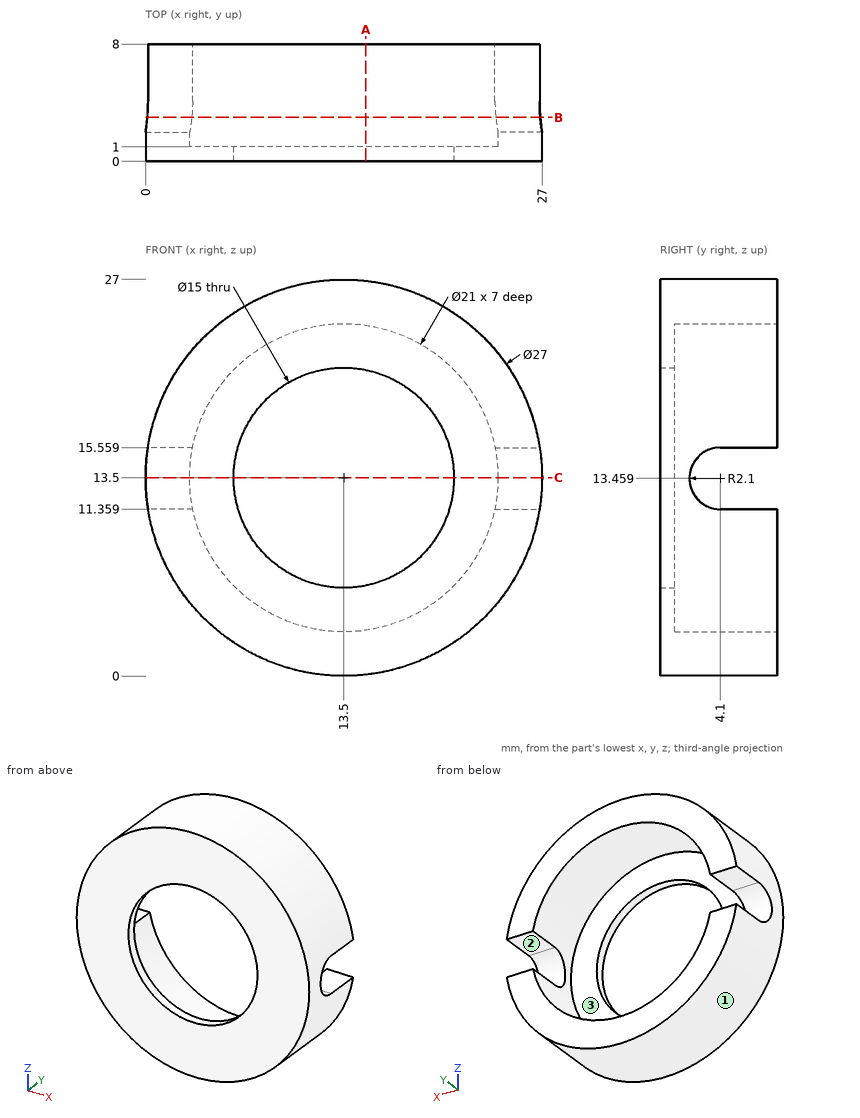
Input: dimensioned drawing with shaded views. Units: mm. Origin: part minimum x, y, z. A direction names the side the tool comes from. Round coordinates to 2 decimals unless told otherwise and drop trailing zeros. Order: outer loops, then holes, each group sorted by start corner. A loop starts at its lowest first (then second) coordinate and runs counter-clockwise, first axis right, second up. Notation, with made-up numbers: (4, 30.25) - (28, 30.25) arc R26 ccw to (28, 57.25) - close; hole circle Ø6 at (18.5, -37.75). An arc over 180 degrees is marked (long way). Use CSV: the item, a comma, the result in double quotes. Start each with the question number.
Q1. First-contact query: pin 1 (6.5 mm diameter, centred on x = 13, z = 18, fed in from +Y); pin 2 (2 mm diameter, centred on y = 2, z = 4.5, fed in from -X); pin 3 (2.5 mm diameter, centred on x = 1.5, y = 6.5, fed in from -Z); pin 4 (5 mm diameter, centred on x = 17.5, z = 4, fed in from +Y). Flat tips, straight axial feed; report the tip coordinate or a pass-through.
Q2. Access query for the marked faces 1, 2 and 3. Directions: +Z, -Z, +X, -X, +Y, -Y. A direction counts if a zero-diameter tool reaches every point of the face in a straight line with its end or side. Return the directions, or none.
Q3. Section query C-C (z = 13.5). Return loops of the section in (x, y).
Q4. Section query A-A (x = 15). Return loops of the section in (y, z).
Q5. Material intervals for line 1 along Z through (x, y) = (13.5, 0.65); line 2 along Z through (x, y) = (13.5, 3.75); line 3 along Y through (x, z) = (14.25, 5), sorted ascending. Write a range as from..to.
Q6. Section query B-B (y = 3). Return loops of the section in (x, z), and give its area (3 significant figures).
Result set:
1,pin 1,"stops at y = 1"
1,pin 2,"stops at x = 2.63"
1,pin 3,"stops at z = 5.33"
1,pin 4,"stops at y = 8"
2,face 1,"+Y, -Y"
2,face 2,"+X, -X, +Y"
2,face 3,"+Y"
3,outline,"(0, 0) - (6, 0) - (6, 1) - (3, 1) - (3, 2) - (0, 2) - close; (21, 0) - (27, 0) - (27, 2) - (24, 2) - (24, 1) - (21, 1) - close"
4,outline,"(0, 0.08) - (8, 0.08) - (8, 3.11) - (1, 3.11) - (1, 6.15) - (0, 6.15) - close; (0, 20.85) - (1, 20.85) - (1, 23.89) - (8, 23.89) - (8, 26.92) - (0, 26.92) - close"
5,line 1,"z = 0..6, 21..27"
5,line 2,"z = 0..3, 24..27"
5,line 3,"y = 0..1"
6,outline,"(0.11, 15.25) - (3.15, 15.25) arc R10.5 cw to (23.85, 15.25) - (26.89, 15.25) arc R13.5 ccw to start; (0.12, 11.67) arc R13.5 ccw to (26.88, 11.67) - (23.84, 11.67) arc R10.5 cw to (3.16, 11.67) - close"
6,area,"205 mm2"
